Source: CAD feature listing. Evaluate the final solid. Frame: model axes, mm. Round coordinates to 2 decimals unless told otherwise and drop trailing zeros. Loops run counter-clockwise (first coordinate to the right, second up) from the corner with the lowest first, then second, coordinate; pieces in that order, holes last.
Item 1: Section query B-B on z = 3. Return loops of the section in (x, y), then the cut area to 3 significant figures.
Item 2: Section query A-A on y = 24. Return loops of the section in (x, z).
Item 3: Ray query, L1, parallel to X at y = 146, z = 6; L2, parallel to Y at x = 13, z = 8; L3, parallel to Y at x = 16.5, z = 4.5. Return the intervals inside material, ascending.
Item 4: Pull-direction query (X, two-part tool) for faces 1 (the flat face through (-3, 170, 5)), 2 (the cylindrical face through (-3.373, 143.315, 4.93)), 3 (the flat face through (-32.776, 84, 5)), 4 (the cylindrical face through (13.748, 126.607, 2.958)); classes: released by +X, released by -X, zero draft, split by the parting line, or undercut.
Item 5: Section query D-D on x = -21. Give the number of separate pieces and of enclosed holes in the cut face, then the cut area to 3 significant figures.
Item 6: First-contact query: P1, Ø11.5, axis at x = 14.72, y = 39, coming from the +Z side; P2, Ø7, axis at x = -20.28, y = 131, coming from the +Z side. Flat tips, straight axial feed; report the tip coordinate or a pass-through.
Item 7: Section query C-C on x = -2. Return loops of the section in (y, z), then the cut area to 3 significant figures.
```python
from build123d import *

# Parameters (mm, degrees)
F0_W     = 60
F0_H     = 170
F0_R     = 4.5
F0_R_2   = 2.75
F1_DEPTH = 10
F2_SIZE  = 4


with BuildPart() as f1:
    # F0 (on Top) → F1 (new body)
    with BuildSketch(Plane.XY):
        with Locations((-2.776433, 85)):
            Rectangle(F0_W, F0_H)
        with Locations((-20.276433, 39)):
            Circle(F0_R, mode=Mode.SUBTRACT)
        with Locations((-2.776433, 24)):
            Circle(F0_R_2, mode=Mode.SUBTRACT)
        with Locations((14.723567, 39)):
            Circle(F0_R, mode=Mode.SUBTRACT)
        with Locations((-20.276433, 131)):
            Circle(F0_R, mode=Mode.SUBTRACT)
        with Locations((-2.776433, 146)):
            Circle(F0_R_2, mode=Mode.SUBTRACT)
        with Locations((14.723567, 131)):
            Circle(F0_R, mode=Mode.SUBTRACT)
    extrude(amount=F1_DEPTH)

    # F2
    f2_edges = [f1.edges().sort_by_distance(p)[0] for p in [
        (-24.776433, 39, 10),
        (10.223567, 39, 10),
        (10.223567, 131, 10),
        (-24.776433, 131, 10),
    ]]
    chamfer(f2_edges, length=F2_SIZE)


solid = f1.part
```
Data:
1. outline: (-32.78, 0) - (27.22, 0) - (27.22, 170) - (-32.78, 170) - close; hole circle Ø9 at (-20.28, 39); hole circle Ø9 at (-20.28, 131); hole circle Ø5.5 at (-2.78, 24); hole circle Ø5.5 at (-2.78, 146); hole circle Ø9 at (14.72, 39); hole circle Ø9 at (14.72, 131)
1. area: 9,900 mm2
2. outline: (-32.78, 0) - (-5.53, 0) - (-5.53, 10) - (-32.78, 10) - close; (-0.03, 0) - (27.22, 0) - (27.22, 10) - (-0.03, 10) - close
3. L1: x = -32.78 to -5.53, -0.03 to 27.22
3. L2: y = 0 to 32.73, 45.27 to 124.73, 137.27 to 170
3. L3: y = 0 to 34.87, 43.13 to 126.87, 135.13 to 170
4. face 1: zero draft
4. face 2: undercut
4. face 3: released by -X
4. face 4: undercut
5. separate pieces: 3
5. enclosed holes: 0
5. area: 1,490 mm2
6. P1: stops at z = 7.25
6. P2: passes through
7. outline: (0, 0) - (21.36, 0) - (21.36, 10) - (0, 10) - close; (26.64, 0) - (143.36, 0) - (143.36, 10) - (26.64, 10) - close; (148.64, 0) - (170, 0) - (170, 10) - (148.64, 10) - close
7. area: 1,590 mm2
